```python
from build123d import *

# Parameters (mm, degrees)
SKETCH_1_W          = 64
SKETCH_1_H          = 64
EXTRUDE_1_DEPTH     = 2
SKETCH_2_R          = 2.05
SKETCH_2_R_2        = 25
CUT_EXTRUDE_1_DEPTH = 2
EXTRUDE_START       = 35
SKETCH_3_R          = 28
SKETCH_3_R_2        = 25
EXTRUDE_2_DEPTH     = 35


with BuildPart() as part:
    # 草图1 → 凸台-拉伸1 (new body)
    with BuildSketch(Plane(origin=(0, 0, 0), x_dir=(1, 0, 0), z_dir=(0, 1, 0))):
        with Locations((8.075949367, -13.283905967)):
            Rectangle(SKETCH_1_W, SKETCH_1_H)
    extrude(amount=EXTRUDE_1_DEPTH)

    # 草图2 → 切除-拉伸1 (cut)
    with BuildSketch(Plane(origin=(0, 2, 0), x_dir=(1, 0, 0), z_dir=(0, 1, 0))):
        with Locations(Location((-16.924050633, 11.716094033, 0), (0, 0, 270))):
            Circle(SKETCH_2_R)
        with Locations(Location((33.075949367, 11.716094033, 0), (0, 0, 270))):
            Circle(SKETCH_2_R)
        with Locations(Location((-16.924050633, -38.283905967, 0), (0, 0, 270))):
            Circle(SKETCH_2_R)
        with Locations(Location((33.075949367, -38.283905967, 0), (0, 0, 270))):
            Circle(SKETCH_2_R)
        with Locations(Location((8.075949367, -13.283905967, 0), (0, 0, 270))):
            Circle(SKETCH_2_R_2)
    extrude(amount=-CUT_EXTRUDE_1_DEPTH, mode=Mode.SUBTRACT)

    # 草图3 → 凸台-拉伸2 (add)
    with BuildSketch(Plane(origin=(0, 2, 0), x_dir=(1, 0, 0), z_dir=(0, 1, 0)).offset(EXTRUDE_START)):
        with Locations(Location((8.075949367, -13.283905967, 0), (0, 0, 270))):
            Circle(SKETCH_3_R)
        with Locations(Location((8.075949367, -13.283905967, 0), (0, 0, 270))):
            Circle(SKETCH_3_R_2, mode=Mode.SUBTRACT)
    extrude(amount=-EXTRUDE_2_DEPTH)


solid = part.part
```
Geometry check sheet. Reference: the model listing, model coordinates, mm. A direction names the side the tool comes from. Give positions to 0.01 mm unless a question says otherwise; leave off trailing zeros. Order: outer loops, then holes, each group sorted by start corner. A loop starts at its lowest first (then second) coordinate and runs counter-clockwise, first axis right, second up. Notation, with made-up numbers: (18, 26.5) -> (58, 26.5) arc R26 cw to (58, 61.5) -> close; hole circle Ø7 at (75, -25.75). An arc over 180 degrees is marked (long way). Write each question's results on one line, items separated by ' | '. Start each with the question number.
(1) Mould release check, pull along Z, two halves, no side actions. Record for faces 1 (the face through (8, 1, 45.284)), 2 (the face through (-18.925, 1.014, 37.84)), 3 (the face through (40.076, 1, 14)): pulls with the +Z half, pulls with the -Z half, needs draft (parallel to the pull), parting line crosses it, or undercut.
(2) Sectioned sample at B-B (z = -0.5). Enter the section's corners in (x, y).
(3) Sectioned sample at A-A (x = -12.5). Enter the section's corners in (y, z).
(4) Sectioned sample at D-D (y = 22.5). Enter the section's corners in (x, z), plus the area to 3 significant figures.
(5) Sectioned sample at C-C (x = 32). Enter the section's corners in (y, z).
(6) Scan lines: line 1 (X direction, y = 32.5, z = 14); line 2 (X direction, y = 31, z = 28.5); line 3 (Y direction, x = 32.5, z = -3). Record each from-to range of solid material in increasing order.
(7) Gauge pin test, flat ends, axial feed: P1, Ø4, axis at y = 21.5, z = 1, coming from the +X side; P2, Ø6.5, axis at x = -16.92, z = -11.72, coming from the +Y side; P3, Ø8, axis at y = 24, z = 9, coming from the +X side. Record the tip position at first contact, or that the pin passes through.
(8) Access from +Z, -Z, +X, -X, +Y, -Y to the whole of each face (thin tool, end or side, straight path). Record for faces 4 (the face through (-21, 2, 13)), 5 (the face through (22, 0, -8)).
Answer below:
1) face 1: pulls with the +Z half | face 2: undercut | face 3: needs draft
2) outline: (-23.92, 0) -> (-12.78, 0) -> (-12.78, 37) -> (-16.3, 37) -> (-16.3, 2) -> (-23.92, 2) -> close; (28.93, 0) -> (40.08, 0) -> (40.08, 2) -> (32.45, 2) -> (32.45, 37) -> (28.93, 37) -> close
3) outline: (0, -18.72) -> (2, -18.72) -> (2, -5.71) -> (37, -5.71) -> (37, -0.92) -> (0, -0.92) -> close; (0, 27.48) -> (37, 27.48) -> (37, 32.27) -> (2, 32.27) -> (2, 45.28) -> (0, 45.28) -> close
4) outline: circle Ø56 at (8.08, 13.28); hole circle Ø50 at (8.08, 13.28) | area: 500 mm2
5) outline: (0, -18.72) -> (2, -18.72) -> (2, -13.46) -> (0, -13.46) -> close; (0, -9.97) -> (2, -9.97) -> (2, -1.26) -> (37, -1.26) -> (37, 6.03) -> (0, 6.03) -> close; (0, 20.54) -> (37, 20.54) -> (37, 27.83) -> (2, 27.83) -> (2, 36.54) -> (0, 36.54) -> close; (0, 40.03) -> (2, 40.03) -> (2, 45.28) -> (0, 45.28) -> close
6) line 1: -19.91 to -16.91, 33.07 to 36.07 | line 2: -15.43 to -11.76, 27.91 to 31.58 | line 3: 0 to 2
7) P1: x = 34.12 | P2: y = 2 | P3: x = 36.07
8) face 4: +Y | face 5: +Z, -Z, +X, -X, -Y
